Can you work these out from the model? Positions are in its coordinate system, mm. A direction names the side the tool comes from. Give positions to 0.01 mm unless a question says otherwise; leave off trailing zeros. Write each loop counter-clockwise with the first axis right and the second up, starting at its lowest first coordinate (ties: lowest second). Pieces come first, ordered by that corner, then holes. Notation, with made-up numbers: (74, -38.5) -> (86, -38.5) arc R18 ccw to (86, -5.5) -> close; hole circle Ø10 at (-23, 66.5). An arc over 180 degrees is marked (long way). One line per item, written item: value.
from build123d import *

# Parameters (mm, degrees)
SKETCH1_W           = 90
SKETCH1_H           = 90
BOSS_EXTRUDE1_DEPTH = 14.3
SKETCH2_W           = 70
SKETCH2_H           = 70
CUT_EXTRUDE1_DEPTH  = 12.6
SKETCH3_R           = 1.725
CUT_EXTRUDE2_DEPTH  = 2.7
CHAMFER1_SIZE       = 5
SKETCH4_R           = 5.5
SKETCH4_R_2         = 1.725
BOSS_EXTRUDE2_DEPTH = 11.8
FILLET1_R           = 2
SKETCH5_R           = 3.25
CUT_EXTRUDE3_DEPTH  = 4
CHAMFER2_SIZE       = 5
CUT_EXTRUDE4_DEPTH  = 13.6


with BuildPart() as part:
    # Sketch1 → Boss-Extrude1 (new body)
    with BuildSketch(Plane(origin=(0, 0, 0), x_dir=(1, 0, 0), z_dir=(0, 1, 0))):
        with Locations((45, 45)):
            Rectangle(SKETCH1_W, SKETCH1_H)
    extrude(amount=BOSS_EXTRUDE1_DEPTH)

    # Sketch2 → Cut-Extrude1 (cut)
    with BuildSketch(Plane(origin=(0, 14.3, 0), x_dir=(1, 0, 0), z_dir=(0, 1, 0))):
        with Locations((45, 45)):
            Rectangle(SKETCH2_W, SKETCH2_H)
    extrude(amount=-CUT_EXTRUDE1_DEPTH, mode=Mode.SUBTRACT)

    # Sketch3 → Cut-Extrude2 (cut, through all)
    with BuildSketch(Plane(origin=(0, 1.7, 0), x_dir=(1, 0, 0), z_dir=(0, 1, 0))):
        with Locations((18.863961034, 18.863961034)):
            Circle(SKETCH3_R)
        with Locations((71.136038966, 71.136038966)):
            Circle(SKETCH3_R)
    extrude(amount=-CUT_EXTRUDE2_DEPTH, mode=Mode.SUBTRACT)

    # Chamfer1
    chamfer1_edges = [part.edges().sort_by_distance(p)[0] for p in [
        (0, 7.15, -90),
        (90, 7.15, -90),
        (90, 7.15, 0),
        (0, 7.15, 0),
    ]]
    chamfer(chamfer1_edges, length=CHAMFER1_SIZE)

    # Sketch4 → Boss-Extrude2 (add)
    with BuildSketch(Plane(origin=(0, 1.7, 0), x_dir=(1, 0, 0), z_dir=(0, 1, 0))):
        with Locations((71.136038966, 71.136038966)):
            Circle(SKETCH4_R)
        with Locations((71.136038966, 71.136038966)):
            Circle(SKETCH4_R_2, mode=Mode.SUBTRACT)
        with Locations((18.863961034, 18.863961034)):
            Circle(SKETCH4_R)
        with Locations((18.863961034, 18.863961034)):
            Circle(SKETCH4_R_2, mode=Mode.SUBTRACT)
    extrude(amount=BOSS_EXTRUDE2_DEPTH)

    # Fillet1
    fillet1_edges = [part.edges().sort_by_distance(p)[0] for p in [
        (65.636038966, 1.7, -71.136038966),
        (13.363961034, 1.7, -18.863961034),
    ]]
    fillet(fillet1_edges, radius=FILLET1_R)

    # Sketch5 → Cut-Extrude3 (cut)
    with BuildSketch(Plane.XZ):
        with Locations((18.863961034, -18.863961034)):
            Circle(SKETCH5_R)
        with Locations((71.136038966, -71.136038966)):
            Circle(SKETCH5_R)
    extrude(amount=-CUT_EXTRUDE3_DEPTH, mode=Mode.SUBTRACT)

    # Chamfer2
    chamfer2_edges = [part.edges().sort_by_distance(p)[0] for p in [
        (10, 8, -10),
        (10, 8, -80),
        (80, 8, -80),
        (80, 8, -10),
    ]]
    chamfer(chamfer2_edges, length=CHAMFER2_SIZE)

    # Sketch6 → Cut-Extrude4 (cut, through all)
    with BuildSketch(Plane(origin=(0, 1.7, 0), x_dir=(1, 0, 0), z_dir=(0, 1, 0))):
        Polygon((80.2, 14.917157288), (80.2, 75.082842712), (75.082842712, 80.2), (14.917157288, 80.2), (9.8, 75.082842712), (9.8, 14.917157288), (14.917157288, 9.8), (75.082842712, 9.8), align=None)
        Polygon((15, 10), (10, 15), (10, 75), (15, 80), (75, 80), (80, 75), (80, 15), (75, 10), align=None, mode=Mode.SUBTRACT)
    extrude(amount=CUT_EXTRUDE4_DEPTH, mode=Mode.SUBTRACT)


solid = part.part
1) Will these pins go through, and if not, where does the flat tip stop? pin 1 (9 mm diameter, centred on x = 72, z = -73.5, fed in from +Y); pin 2 (2 mm diameter, centred on x = 18, z = -19.5, fed in from -Y); pin 3 (1.5 mm diameter, centred on x = 54.5, z = -35.5, fed in from +Y); pin 4 (3 mm diameter, centred on x = 71.14, z = -71.14, fed in from -Y).
Answer list:
pin 1: stops at y = 13.5
pin 2: stops at y = 4
pin 3: stops at y = 1.7
pin 4: passes through
2) For faces 4 (the face through (18.148, 8.531, -24.317)), 5 (the face through (19.79, 8.68, -20.32)), 6 (the face through (20.3, 4, -20.3)), which set-ups out of +Z, -Z, +X, -X, +Y, -Y let a thin tool reach every point of the face, with its end or its side?
Answer list:
face 4: +Y
face 5: +Y, -Y
face 6: -Y
3) If we section it at B-B (x = 36): Write out the boundary of the cut face in (y, z).
Answer list:
outline: (0, -90) -> (14.3, -90) -> (14.3, -80.2) -> (1.7, -80.2) -> (1.7, -9.8) -> (14.3, -9.8) -> (14.3, 0) -> (0, 0) -> close
4) If we section it at C-C (z = -51): Write out the boundary of the cut face in (x, y).
Answer list:
outline: (0, 0) -> (90, 0) -> (90, 14.3) -> (80.2, 14.3) -> (80.2, 1.7) -> (9.8, 1.7) -> (9.8, 14.3) -> (0, 14.3) -> close
5) If we section it at A-A (y = 7.5): Write out the boundary of the cut face in (x, z) (3 decimals), and give its area (3 significant figures).
Answer list:
outline: (0, -85) -> (5, -90) -> (85, -90) -> (90, -85) -> (90, -5) -> (85, 0) -> (5, 0) -> (0, -5) -> close; circle Ø11 at (18.864, -18.864); circle Ø11 at (71.136, -71.136); hole (9.8, -75.083) -> (14.917, -80.2) -> (75.083, -80.2) -> (80.2, -75.083) -> (80.2, -14.917) -> (75.083, -9.8) -> (14.917, -9.8) -> (9.8, -14.917) -> close; hole circle Ø3.45 at (18.864, -18.864); hole circle Ø3.45 at (71.136, -71.136)
area: 3,320 mm^2
6) We'd pull the mould along Z, two halves only. Please class faces 1 (the face through (74, 13.5, -71)), 2 (the face through (44, 0, -46)), 3 (the face through (88, 7, -3)): released by +Z, released by -Z, zero draft, split by the parting line, or undercut.
Answer list:
face 1: undercut
face 2: zero draft
face 3: released by +Z
7) I need wall thicknesses on L1, parallel to Z at x = 34, y = 12.75; L2, parallel to Z at x = 68, y = 6; L3, parallel to Z at x = 67, y = 3.25. Which ranges of each line are inside material? Lowest first, please.
Answer list:
L1: z = -90 to -80.2, -9.8 to 0
L2: z = -90 to -80.2, -75.65 to -66.62, -9.8 to 0
L3: z = -90 to -80.2, -74.84 to -67.43, -9.8 to 0
